The drawing under review shows one solid part. Ordinate dimensions are in mm from its lowest x, y, z. Give positions to 0.01 mm unless a question says otherwise; leave off trailing zeros. Write each loop counter-clockwise with the first axis right and the second up, starting at its lowest first coordinate (ties: lowest second). Pieces come first, ordered by that corner, then holes. Notation, with made-up numbers: (-29.75, 11.25) -> (16.25, 11.25) arc R18 ccw to (16.25, 28.25) -> close; hole circle Ø11 at (5.5, 74.5). An arc over 180 degrees is marked (long way). Answer as a JSON object with one key per item and string values.
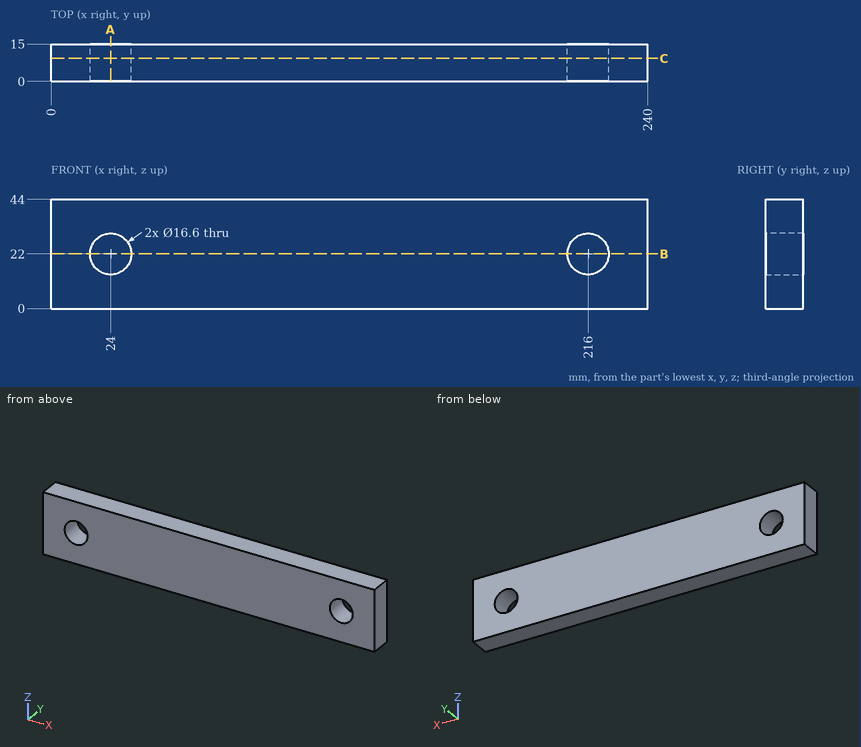
(1) We need section C-C, the plane y = 9.25. State the section outline as (x, z) points, then the cut area to 3 significant figures.
Here are the results:
{"outline": "(0, 0) -> (240, 0) -> (240, 44) -> (0, 44) -> close; hole circle Ø16.6 at (24, 22); hole circle Ø16.6 at (216, 22)", "area": "10,100 mm²"}
(2) We need section B-B, the plane z = 22. State the section outline as (x, y) points.
Here are the results:
{"outline": "(0, 0) -> (15.7, 0) -> (15.7, 15) -> (0, 15) -> close; (32.3, 0) -> (207.7, 0) -> (207.7, 15) -> (32.3, 15) -> close; (224.3, 0) -> (240, 0) -> (240, 15) -> (224.3, 15) -> close"}
(3) Clearance check with a flat-ended pin moving along its axis: pin 1 (13.5 mm diameter, centred on x = 216, z = 22, fed in from -Y). State where the tip first meets the part, or that it passes through.
Here are the results:
{"pin 1": "passes through"}
(4) We need section A-A, the plane x = 24. State the section outline as (y, z) points, then the cut area to 3 significant figures.
Here are the results:
{"outline": "(0, 0) -> (15, 0) -> (15, 13.7) -> (0, 13.7) -> close; (0, 30.3) -> (15, 30.3) -> (15, 44) -> (0, 44) -> close", "area": "411 mm²"}
(5) For line 1 along X through (y, z) = (12.25, 22); line 2 along X through (y, z) = (3, 24); line 3 along Z through (x, y) = (17, 7.25), list the stretches that pass through material, from the lowest coordinate up.
Here are the results:
{"line 1": "x = 0 to 15.7, 32.3 to 207.7, 224.3 to 240", "line 2": "x = 0 to 15.94, 32.06 to 207.94, 224.06 to 240", "line 3": "z = 0 to 17.54, 26.46 to 44"}
